Check sheet for the modelled part. Datum: model origin and axes. Units: mm. Face numbers are marked on the shaded views. Round coordinates to 2 decimals unless told otherwise and drop trailing zeros. Write each loop counter-clockwise with the first axis right and the second up, starting at its lowest first coordinate (ties: lowest second). Pieces come first, ordered by that corner, then holes. Notation, with made-up numbers: (45.5, 16) -> (103.5, 16) arc R24 ccw to (103.5, 52) -> close; hole circle Ø11 at (23, 71). An arc over 180 degrees is marked (long way). One line per item, written item: value. Start each with the question number.
```python
from build123d import *

# Parameters (mm, degrees)
CROQUIS1_W              = 200
CROQUIS1_H              = 75.4
CROQUIS1_R              = 25.4
SALIENTE_EXTRUIR1_DEPTH = 12.7
CROQUIS2_R              = 7.14375
CORTAR_EXTRUIR1_DEPTH   = 15


with BuildPart() as part:
    # Croquis1 → Saliente-Extruir1 (new body)
    with BuildSketch(Plane.XY):
        with Locations((0, -12.3)):
            Rectangle(CROQUIS1_W, CROQUIS1_H)
        with Locations((0, -12.3)):
            Circle(CROQUIS1_R, mode=Mode.SUBTRACT)
    extrude(amount=SALIENTE_EXTRUIR1_DEPTH)

    # Croquis2 → Cortar-Extruir1 (cut)
    with BuildSketch(Plane.XY.offset(12.7)):
        with Locations((-70, 5.7)):
            Circle(CROQUIS2_R)
        with Locations((-70, -30.3)):
            Circle(CROQUIS2_R)
        with Locations((70, -30.3)):
            Circle(CROQUIS2_R)
        with Locations((70, 5.7)):
            Circle(CROQUIS2_R)
    extrude(amount=-CORTAR_EXTRUIR1_DEPTH, mode=Mode.SUBTRACT)


solid = part.part
```
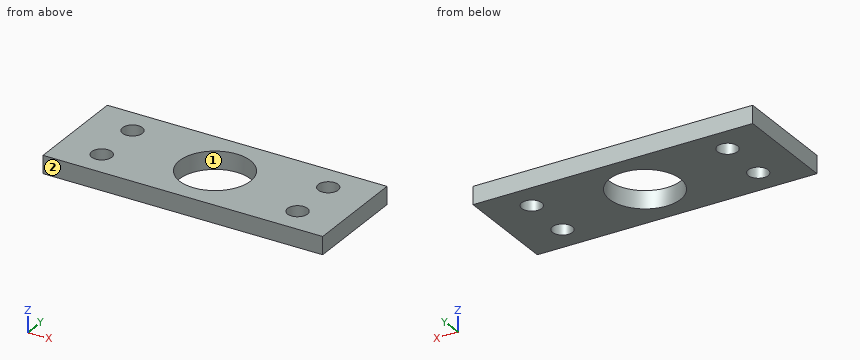
1. Cross-section at C-C (y = 5.7). Record the cut outline in (x, z), plus the area to 3 significant figures.
2. Material ranges on probe 1 along Y at (x, z) = (-70, 6); probe 2 along X at (y, z) = (-24, 9.25); probe 3 along Y at (x, z) = (-76, 9.75), recorded low to high.
3. Depth check by flat-ended pin: pin 1 Ø12 at (x, y) = (70, -26.5) entering from +Z. Enter the tip coordinate at first touch or a pass-through.
4. Release check for a two-part mould opening along X. For the marked faces 1 and 2 record: +X half, -X half, draft (parallel to the pull), parting line (faces both ways), or undercut.
5. Cross-section at D-D (x = -13.5). Record the cut outline in (y, z), plus the area to 3 significant figures.
6. Cross-section at B-B (x = 70). Record the cut outline in (y, z), plus the area to 3 significant figures.
7. Cross-section at A-A (z = 5). Record the cut outline in (x, y), plus the area to 3 significant figures.
Working result:
1. outline: (-100, 0) -> (-77.14, 0) -> (-77.14, 12.7) -> (-100, 12.7) -> close; (-62.86, 0) -> (-17.92, 0) -> (-17.92, 12.7) -> (-62.86, 12.7) -> close; (17.92, 0) -> (62.86, 0) -> (62.86, 12.7) -> (17.92, 12.7) -> close; (77.14, 0) -> (100, 0) -> (100, 12.7) -> (77.14, 12.7) -> close
1. area: 1,720 mm^2
2. probe 1: y = -50 to -37.44, -23.16 to -1.44, 12.84 to 25.4
2. probe 2: x = -100 to -73.37, -66.63 to -22.54, 22.54 to 66.63, 73.37 to 100
2. probe 3: y = -50 to -34.18, -26.42 to 1.82, 9.58 to 25.4
3. pin 1: stops at z = 12.7
4. face 1: undercut
4. face 2: draft
5. outline: (-50, 0) -> (-33.82, 0) -> (-33.82, 12.7) -> (-50, 12.7) -> close; (9.22, 0) -> (25.4, 0) -> (25.4, 12.7) -> (9.22, 12.7) -> close
5. area: 411 mm^2
6. outline: (-50, 0) -> (-37.44, 0) -> (-37.44, 12.7) -> (-50, 12.7) -> close; (-23.16, 0) -> (-1.44, 0) -> (-1.44, 12.7) -> (-23.16, 12.7) -> close; (12.84, 0) -> (25.4, 0) -> (25.4, 12.7) -> (12.84, 12.7) -> close
6. area: 595 mm^2
7. outline: (-100, -50) -> (100, -50) -> (100, 25.4) -> (-100, 25.4) -> close; hole circle Ø14.29 at (-70, -30.3); hole circle Ø14.29 at (-70, 5.7); hole circle Ø50.8 at (0, -12.3); hole circle Ø14.29 at (70, -30.3); hole circle Ø14.29 at (70, 5.7)
7. area: 12,400 mm^2
